```python
from build123d import *

# Parameters (mm, degrees)
SKETCH1_R           = 265.7
SKETCH1_R_2         = 211.5
SKETCH1_R_3         = 20
SKETCH1_R_4         = 5
EXTRUDE1_DEPTH      = 5
SKETCH2_R           = 265.7
SKETCH2_R_2         = 15
SKETCH2_R_3         = 211.5
EXTRUDE2_DEPTH      = 25
SKETCH3_R           = 265.7
SKETCH3_R_2         = 260.7
EXTRUDE3_DEPTH      = 200
SKETCH4_R           = 311
EXTRUDE4_DEPTH      = 266.7
EXTRUDE4_DEPTH_BACK = 266.7


with BuildPart() as part:
    # Sketch1 → Extrude1 (new body)
    with BuildSketch(Plane.XY):
        Circle(SKETCH1_R)
        Circle(SKETCH1_R_2, mode=Mode.SUBTRACT)
        with Locations((238.6, 0)):
            Circle(SKETCH1_R_3, mode=Mode.SUBTRACT)
        with Locations((168.715677991, 168.715677991)):
            Circle(SKETCH1_R_3, mode=Mode.SUBTRACT)
        with Locations((0, 238.6)):
            Circle(SKETCH1_R_3, mode=Mode.SUBTRACT)
        with Locations((-168.715677991, 168.715677991)):
            Circle(SKETCH1_R_3, mode=Mode.SUBTRACT)
        with Locations((-238.6, 0)):
            Circle(SKETCH1_R_3, mode=Mode.SUBTRACT)
        with Locations((-168.715677991, -168.715677991)):
            Circle(SKETCH1_R_3, mode=Mode.SUBTRACT)
        with Locations((0, -238.6)):
            Circle(SKETCH1_R_3, mode=Mode.SUBTRACT)
        with Locations((168.715677991, -168.715677991)):
            Circle(SKETCH1_R_3, mode=Mode.SUBTRACT)
        with Locations((230.469902153, 61.754224161)):
            Circle(SKETCH1_R_4, mode=Mode.SUBTRACT)
        with Locations((-230.469902153, 61.754224161)):
            Circle(SKETCH1_R_4, mode=Mode.SUBTRACT)
        with Locations((-91.308266962, -220.437656457)):
            Circle(SKETCH1_R_4, mode=Mode.SUBTRACT)
    extrude(amount=EXTRUDE1_DEPTH)

    # Sketch2 → Extrude2 (add)
    with BuildSketch(Plane.XY.offset(5)):
        Circle(SKETCH2_R)
        with Locations((238.6, 0)):
            Circle(SKETCH2_R_2, mode=Mode.SUBTRACT)
        with Locations((168.715677991, 168.715677991)):
            Circle(SKETCH2_R_2, mode=Mode.SUBTRACT)
        with Locations((0, 238.6)):
            Circle(SKETCH2_R_2, mode=Mode.SUBTRACT)
        with Locations((-168.715677991, 168.715677991)):
            Circle(SKETCH2_R_2, mode=Mode.SUBTRACT)
        with Locations((-238.6, 0)):
            Circle(SKETCH2_R_2, mode=Mode.SUBTRACT)
        with Locations((-168.715677991, -168.715677991)):
            Circle(SKETCH2_R_2, mode=Mode.SUBTRACT)
        with Locations((0, -238.6)):
            Circle(SKETCH2_R_2, mode=Mode.SUBTRACT)
        with Locations((168.715677991, -168.715677991)):
            Circle(SKETCH2_R_2, mode=Mode.SUBTRACT)
        Circle(SKETCH2_R_3, mode=Mode.SUBTRACT)
    extrude(amount=EXTRUDE2_DEPTH)

    # Sketch3 → Extrude3 (add)
    with BuildSketch(Plane.XY.offset(30)):
        Circle(SKETCH3_R)
        Circle(SKETCH3_R_2, mode=Mode.SUBTRACT)
    extrude(amount=EXTRUDE3_DEPTH)

    # Sketch4 → Extrude4 (cut, two sides)
    with BuildSketch(Plane(origin=(0, 0, 0), x_dir=(0, 0, -1), z_dir=(1, 0, 0))) as extrude4_sk:
        with Locations((-400, 0)):
            Circle(SKETCH4_R)
    extrude(amount=EXTRUDE4_DEPTH, mode=Mode.SUBTRACT)
    extrude(extrude4_sk.sketch, amount=-EXTRUDE4_DEPTH_BACK, mode=Mode.SUBTRACT)


solid = part.part
```
Here's how the part is built. I have some questions about the finished solid (model axes, mm). A direction names the side the tool comes from. Give positions to 0.01 mm unless a question says otherwise; leave off trailing zeros. Order: outer loops, then holes, each group sorted by start corner. A loop starts at its lowest first (then second) coordinate and runs counter-clockwise, first axis right, second up. Notation, with made-up numbers: M -9,52.5 L 36,52.5 A33 cw 36,91.5 Z; hole C 28,66.25 d10. An arc over 180 degrees is marked long. Use a Markdown table: item, result. Add a question column.
1. Suppose I cut it at B-B (z = 131). List the corners of the cut face in (x, y) for me.
2. For pin 1 Ø2 at (x, z) = (2, 166.5) entering from -Y; pin 2 Ø11.5 at (x, y) = (-91.31, -220.44) entering from -Z; pin 3 Ø5 at (x, y) = (-89.5, -220.5) entering from -Z; pin 4 Ø5 at (x, z) = (-199.5, 95.5) entering from +Y, each with a flat end and sliding along its axis, tell me the tip position at first contact or that it passes through.
3. On a 3-axis mill with a long thin cutter (end or side, diameter ignored), from which of +Z, -Z, +X, -X, +Y, -Y can I reach the whole of each face in a straight line? I mean faces 1 (the cylindrical face through (6.92, -251.91, 17.32)), 2 (the cylindrical face through (152.84, 156.55, 2.46)), 3 (the flat face through (211, -18, 30)). Say none if no direction works.
4. Suppose I cut it at C-C (y = 41.5). List the corners of the cut face in (x, z) for me, and give its area (3 significant figures).
5. Suppose I cut it at A-A (x = 0). List the corners of the cut face in (y, z) for me, and give its area (3 significant figures).
6. Suppose I cut it at D-D (x = -119). List the corners of the cut face in (y, z) for me, and give its area (3 significant figures).
7. I need wall thicknesses on probe 1 along Y at (x, z) = (0, 15.75); probe 2 along Z at (x, y) = (-182.5, 145.5); probe 3 along X at (y, z) = (233, 172.5). Which ranges of each line are inside material? Lowest first, please. Write a range as from..to.
Results list:
| question | item | result |
|---|---|---|
| 1 | outline | M -215.03,-156.08 A265.7 ccw 215.03,-156.08 L 208.82,-156.08 A260.7 cw -208.82,-156.08 Z; M -215.03,156.08 L -208.82,156.08 A260.7 cw 208.82,156.08 L 215.03,156.08 A265.7 ccw Z |
| 2 | pin 1 | stops at y = -265.7 |
| 2 | pin 2 | stops at z = 0 |
| 2 | pin 3 | stops at z = 5 |
| 2 | pin 4 | stops at y = 178.29 |
| 3 | face 1 | +Z, -Z |
| 3 | face 2 | -Z |
| 3 | face 3 | +Z |
| 4 | outline | M -262.44,0 L -207.39,0 L -207.39,30 L -257.38,30 L -257.38,91.78 L -262.44,91.78 Z; M 207.39,0 L 262.44,0 L 262.44,91.78 L 257.38,91.78 L 257.38,30 L 207.39,30 Z |
| 4 | area | 3,930 mm² |
| 5 | outline | M -265.7,0 L -258.6,0 L -258.6,5 L -253.6,5 L -253.6,30 L -260.7,30 L -260.7,230 L -265.7,230 Z; M -223.6,5 L -218.6,5 L -218.6,0 L -211.5,0 L -211.5,30 L -223.6,30 Z; M 211.5,0 L 218.6,0 L 218.6,5 L 223.6,5 L 223.6,30 L 211.5,30 Z; M 253.6,5 L 258.6,5 L 258.6,0 L 265.7,0 L 265.7,230 L 260.7,230 L 260.7,30 L 253.6,30 Z |
| 5 | area | 3,350 mm² |
| 6 | outline | M -237.56,0 L -174.85,0 L -174.85,30 L -231.96,30 L -231.96,192.83 A311 cw -237.56,199.29 Z; M 174.85,0 L 237.56,0 L 237.56,199.29 A311 cw 231.96,192.83 L 231.96,30 L 174.85,30 Z |
| 6 | area | 5,620 mm² |
| 7 | probe 1 | y = -265.7..-253.6, -223.6..-211.5, 211.5..223.6, 253.6..265.7 |
| 7 | probe 2 | z = 0..30 |
| 7 | probe 3 | x = -127.7..-116.94, 116.94..127.7 |
